Input: part model. Units: mm. Frame: model coordinates. Face numbers are marked on the shaded views. A direction names the side the tool comes from. Coordinates: 2 decimals unless noted, no trailing zeros. Write each loop counter-clockwise with the first axis right and the second up, starting at its lowest first coordinate (ties: lowest second). Pieces come first, ordered by that corner, then holes. Notation, with made-up numbers: (56.25, 36.25) - (60.25, 36.25) arc R24 cw to (60.25, 54.25) - close; hole circle Ø1 at (39, 49). An arc over 180 degrees is marked (long way). Use a Markdown table: item, result. Add a question column.
Q1. Set-up query: the marked faces 1 and 2. Return all of +Z, -Z, +X, -X, +Y, -Y with unobstructed straight access to the full face (end or side cutting, diameter ignored); none if empty.
Q2. Mould query, pull axis Y, two halves, no side actions, for the marked faces 3, 4, 5 and 6. Classes: released by +Y, released by -Y, zero draft, split by the parting line, or undercut.
Q3. Section query A-A (z = -1.75). Return the cut outline in (x, y).
Q4. Pin query (flat end, axial travel): P1, Ø0.6, axis at x = 1, z = -3, coming from the +Y side; P2, Ø9.5, axis at y = 9, z = 3, coming from the +X side; P3, Ø9.5, axis at y = 11.5, z = 3.5, coming from the -X side. Return the tip coordinate at first contact, or that it passes through.
Q5. Material intervals for probe 1 along X at (y, z) = (-14, 7.5); probe 2 along Y at (x, z) = (-3, 0.25) (3 decimals); probe 3 along Y at (x, z) = (-6.25, 8), sorted ascending. Write a range as from..to.
Q6. Section query C-C (y = -67.5). Return the cut outline in (x, z).
Q7. Section query B-B (x = -8.75). Return the cut outline in (y, z), then the cut area to 3 significant figures.
from build123d import *

# Parameters (mm, degrees)
F1_DEPTH = 9
F2_R     = 5
F4_START = -10
F4_DEPTH = 20
F6_DEPTH = 10
F7_R     = 5


with BuildPart() as f1:
    # F0 (on Top) → F1 (new body, symmetric)
    with BuildSketch(Plane.XY):
        with BuildLine():
            Line((-2.6, 2.2), (0, -7.5033320997))
            Line((0, -7.5033320997), (0, -129.5))
            ThreePointArc((0, -129.5), (-7.1872847082, -137.4586113019), (-15.8348734636, -131.1170212766))
            ThreePointArc((-15.8348734636, -131.1170212766), (-17.3482014958, -130.0072430222), (-18.6059763198, -131.4))
            ThreePointArc((-18.6059763198, -131.4), (-12.7073180305, -145.995204112), (1.6758691731, -152.3934912697))
            ThreePointArc((1.6758691731, -152.3934912697), (2.1863683898, -152.1973413167), (2.4, -151.6939073197))
            Line((2.4, -151.6939073197), (2.4, 1.5))
            ThreePointArc((2.4, 1.5), (2.1949747468, 1.9949747468), (1.7, 2.2))
            Line((1.7, 2.2), (0.5, 2.2))
            ThreePointArc((0.5, 2.2), (0.0050252532, 2.4050252532), (-0.2, 2.9))
            Line((-0.2, 2.9), (-0.2, 15))
            Line((-0.2, 15), (-2.6, 15))
            Line((-2.6, 15), (-2.6, 2.2))
        make_face()
    extrude(amount=F1_DEPTH, both=True)

    # F2
    f2_edges = [f1.edges().sort_by_distance(p)[0] for p in [
        (-2.6, 2.2, 0),
        (0, -7.503332, 0),
    ]]
    fillet(f2_edges, radius=F2_R)

    # F3 (on Right) → F4 (cut)
    with BuildSketch(Plane.YZ.offset(F4_START)):
        with BuildLine():
            ThreePointArc((-129.4, -5), (-130.5715728753, -7.8284271247), (-133.4, -9))
            Line((-133.4, -9), (-133.4, -10))
            Line((-133.4, -10), (-128.4, -10))
            Line((-128.4, -10), (-128.4, 10))
            Line((-128.4, 10), (-133.4, 10))
            Line((-133.4, 10), (-133.4, 9))
            ThreePointArc((-133.4, 9), (-130.5715728753, 7.8284271247), (-129.4, 5))
            Line((-129.4, 5), (-129.4, -5))
        make_face()
    extrude(amount=-F4_DEPTH, mode=Mode.SUBTRACT)

    # F5 (on Right) → F6 (cut)
    with BuildSketch(Plane.YZ):
        with BuildLine():
            ThreePointArc((7.7, -5.25), (7.9121320344, -5.1621320344), (8, -4.95))
            Line((8, -4.95), (8, 4.95))
            ThreePointArc((8, 4.95), (7.9121320344, 5.1621320344), (7.7, 5.25))
            Line((7.7, 5.25), (5.5, 5.25))
            ThreePointArc((5.5, 5.25), (4.7928932188, 4.9571067812), (4.5, 4.25))
            Line((4.5, 4.25), (4.5, -4.25))
            ThreePointArc((4.5, -4.25), (4.7928932188, -4.9571067812), (5.5, -5.25))
            Line((5.5, -5.25), (7.7, -5.25))
        make_face()
    extrude(amount=-F6_DEPTH, mode=Mode.SUBTRACT)

    # F7
    f7_edges = [f1.edges().sort_by_distance(p)[0] for p in [
        (-1.4, 15, -9),
        (-1.4, 15, 9),
    ]]
    fillet(f7_edges, radius=F7_R)


solid = f1.part
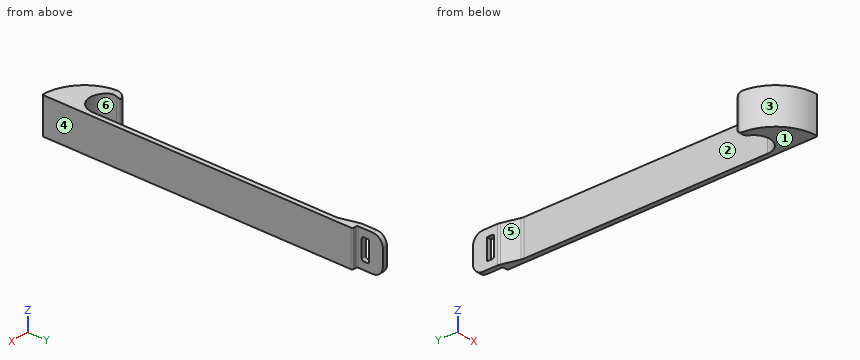
Values follow:
| question | item | result |
|---|---|---|
| 1 | face 1 | -Z, +X, -X, +Y, -Y |
| 1 | face 2 | +Z, -Z, -X |
| 2 | face 3 | released by -Y |
| 2 | face 4 | zero draft |
| 2 | face 5 | undercut |
| 2 | face 6 | undercut |
| 3 | outline | (-18.61, -131.4) arc R21.01 ccw to (1.68, -152.39) arc R0.7 ccw to (2.4, -151.69) - (2.4, 1.5) arc R0.7 ccw to (1.7, 2.2) - (0.5, 2.2) arc R0.7 cw to (-0.2, 2.9) - (-0.2, 4.5) - (-2.6, 4.5) - (-2.6, 2.86) arc R5 ccw to (-2.43, 1.56) - (-0.17, -6.87) arc R5 cw to (0, -8.16) - (0, -129.5) arc R8 cw to (-15.83, -131.12) arc R1.4 ccw to start; (-2.6, 8) - (-0.2, 8) - (-0.2, 15) - (-2.6, 15) - close |
| 4 | P1 | y = 2.2 |
| 4 | P2 | x = -0.2 |
| 4 | P3 | x = -2.6 |
| 5 | probe 1 | 0..2.4 |
| 5 | probe 2 | -151.7..-135.745 |
| 5 | probe 3 | -150.54..-137.31 |
| 6 | outline | (0, -9) - (2.4, -9) - (2.4, 9) - (0, 9) - close |
| 7 | outline | (-149.2, -9) - (-137.46, -9) - (-137.46, 9) - (-149.2, 9) - close |
| 7 | area | 211 mm2 |
